Part model, mm, in its own coordinate system. Face numbers are marked on the shaded views. A direction names the side the tool comes from. Coordinates: 2 decimals unless noted, no trailing zeros. Write each loop counter-clockwise with the first axis right and the second up, starting at its lowest first coordinate (ties: lowest second). Pieces come first, ordered by that corner, then holes. Notation, with made-up numbers: (46.25, 25) - (53.25, 25) arc R24 ccw to (53.25, 45) - close; hole circle Ø11 at (28, 72.25). An arc over 180 degrees is marked (long way). Write each question's results on one line, items separated by ' | '.
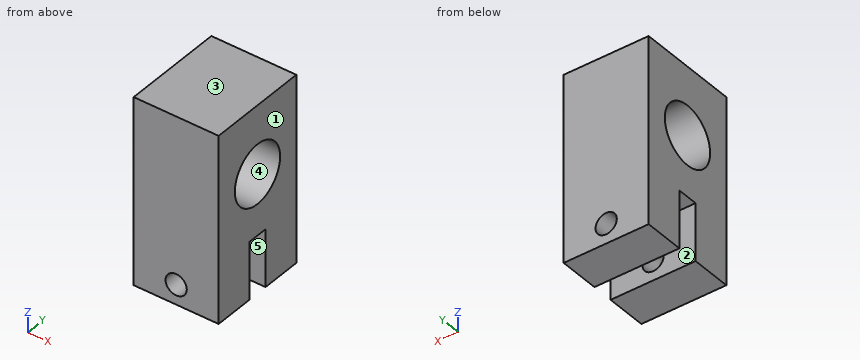
from build123d import *

# Parameters (mm, degrees)
SKETCH_1_R          = 7
EXTRUDE_1_DEPTH     = 20
SKETCH_2_R          = 2.5
CUT_EXTRUDE_2_DEPTH = 42.896701285


with BuildPart() as part:
    # Эскиз1 → Вытянуть1 (new body)
    with BuildSketch(Plane(origin=(0, 0, 0), x_dir=(0, 0, -1), z_dir=(1, 0, 0))):
        Polygon((-16.093397181, 12), (27.91654668, 12), (27.91654668, 2.5), (14.371474957, 2.5), (14.371474957, -2.5), (27.91654668, -2.5), (27.91654668, -12), (-16.093397181, -12), align=None)
        Circle(SKETCH_1_R, mode=Mode.SUBTRACT)
    extrude(amount=EXTRUDE_1_DEPTH)

    # Эскиз2 → Вытянуть2 (cut, through all)
    with BuildSketch(Plane(origin=(0, 12, 0), x_dir=(1, 0, 0), z_dir=(0, 1, 0))):
        with Locations(Location((10, 23.262831067, 0), (0, 0, 270))):
            Circle(SKETCH_2_R)
    extrude(amount=-CUT_EXTRUDE_2_DEPTH, mode=Mode.SUBTRACT)


solid = part.part
(1) Saw through at C-C on y = 0. Write the cut outline in (x, z).
Return value:
outline: (0, -14.37) - (20, -14.37) - (20, -7) - (0, -7) - close; (0, 7) - (20, 7) - (20, 16.09) - (0, 16.09) - close
(2) Saw through at A-A on z = -15. Write the cut outline in (x, y).
Return value:
outline: (0, -12) - (20, -12) - (20, -2.5) - (0, -2.5) - close; (0, 2.5) - (20, 2.5) - (20, 12) - (0, 12) - close
(3) 3-axis set-ups, long thin cutter, end or side, ignore diameter. For the marked faces 1 and 2: which of +Z, -Z, +X, -X, +Y, -Y reach the whole face in a straight line?
Return value:
face 1: +Z, -Z, +X, +Y, -Y | face 2: -Z, +X, -X
(4) Two-plate mould, pull along Z, no slides. Class the marked faces 3, 4 and 5: released by +Z, released by -Z, zero draft, split by the parting line, or undercut.
Return value:
face 3: released by +Z | face 4: undercut | face 5: zero draft
(5) Wall check: line 1 (Y direction, x = 18.75, z = -24); line 2 (Z direction, x = 4, y = 1.5); line 3 (Y direction, x = 10.5, z = 1). Give the ranges that are in metal, low to high. Write a range as from..to.
Return value:
line 1: y = -12..-2.5, 2.5..12 | line 2: z = -14.37..-6.84, 6.84..16.09 | line 3: y = -12..-6.93, 6.93..12
(6) Flat gauge pin, fed straight in: P1, Ø4.5, axis at x = 10, z = -23.26, coming from the +Y side. Where does the tip first touch, or does it go through?
Return value:
P1: passes through
(7) Saw through at D-D on x = 5.5. Write the cut outline in (y, z).
Return value:
outline: (-12, -27.92) - (-2.5, -27.92) - (-2.5, -14.37) - (2.5, -14.37) - (2.5, -27.92) - (12, -27.92) - (12, 16.09) - (-12, 16.09) - close; hole circle Ø14 at (0, 0)
(8) Saw through at B-B on x = 10. Write the cut outline in (y, z).
Return value:
outline: (-12, -27.92) - (-2.5, -27.92) - (-2.5, -25.76) - (-12, -25.76) - close; (-12, -20.76) - (-2.5, -20.76) - (-2.5, -14.37) - (2.5, -14.37) - (2.5, -20.76) - (12, -20.76) - (12, 16.09) - (-12, 16.09) - close; (2.5, -27.92) - (12, -27.92) - (12, -25.76) - (2.5, -25.76) - close; hole circle Ø14 at (0, 0)
